from build123d import *

# Parameters (mm, degrees)
BOSS_EXTRUDE2_DEPTH = 1.6
CUT_EXTRUDE3_START  = 1.6
SKETCH1_R           = 0.5
CUT_EXTRUDE3_DEPTH  = 47.684310176
CUT_EXTRUDE4_START  = 1.6
SKETCH3_R           = 1
CUT_EXTRUDE4_DEPTH  = 1.6
FILLET1_R           = 1


with BuildPart() as part:
    # Sketch2 → Boss-Extrude2 (new body)
    with BuildSketch(Plane.XY):
        with BuildLine():
            Line((-16.263194882, -20.445638098), (-23.811184851, -29.934762))
            ThreePointArc((-23.811184851, -29.934762), (0, -38.25), (23.811184851, -29.934762))
            Line((23.811184851, -29.934762), (16.263194882, -20.445638098))
            ThreePointArc((16.263194882, -20.445638098), (0, -26.125), (-16.263194882, -20.445638098))
        make_face()
    extrude(amount=BOSS_EXTRUDE2_DEPTH)

    # Sketch1 → Cut-Extrude3 (cut, through all)
    with BuildSketch(Plane.XY.offset(CUT_EXTRUDE3_START)):
        with Locations((-15.454132619, -23.797277365)):
            Circle(SKETCH1_R)
        with Locations((-12.88198043, -25.282310124)):
            Circle(SKETCH1_R)
        with Locations((-10.168690568, -26.490344602)):
            Circle(SKETCH1_R)
        with Locations((-7.343990405, -27.408145321)):
            Circle(SKETCH1_R)
        with Locations((-4.438827946, -28.025656664)):
            Circle(SKETCH1_R)
        with Locations((-1.485032758, -28.336113049)):
            Circle(SKETCH1_R)
        with Locations((1.485032758, -28.336113049)):
            Circle(SKETCH1_R)
        with Locations((4.438827946, -28.025656664)):
            Circle(SKETCH1_R)
        with Locations((7.343990405, -27.408145321)):
            Circle(SKETCH1_R)
        with Locations((10.168690568, -26.490344602)):
            Circle(SKETCH1_R)
        with Locations((12.88198043, -25.282310124)):
            Circle(SKETCH1_R)
        with Locations((15.454132619, -23.797277365)):
            Circle(SKETCH1_R)
    extrude(amount=-CUT_EXTRUDE3_DEPTH, mode=Mode.SUBTRACT)

    # Sketch3 → Cut-Extrude4 (cut)
    with BuildSketch(Plane.XY.offset(CUT_EXTRUDE4_START)):
        with Locations((-17.6875, -30.635648659)):
            Circle(SKETCH3_R)
        with Locations((17.6875, -30.635648659)):
            Circle(SKETCH3_R)
    extrude(amount=-CUT_EXTRUDE4_DEPTH, mode=Mode.SUBTRACT)

    # Fillet1
    fillet1_edges = [part.edges().sort_by_distance(p)[0] for p in [
        (16.263194882, -20.445638098, 0.8),
        (23.811184851, -29.934762, 0.8),
        (-23.811184851, -29.934762, 0.8),
        (-16.263194882, -20.445638098, 0.8),
    ]]
    fillet(fillet1_edges, radius=FILLET1_R)


solid = part.part
The listing builds one solid part. Answer for the finished solid, in the listing's coordinates (mm). Round coordinates to 2 decimals unless told otherwise and drop trailing zeros. Loops run counter-clockwise (first coordinate to the right, second up) from the corner with the lowest first, then second, coordinate; pieces in that order, holes last. Notation, with made-up numbers: M 62.25,49.5 L 73.25,49.5 A22 cw 73.25,67.5 Z; hole C 83.25,9 d8. An arc over 180 degrees is marked long. Return JSON: item names as keys, results as strings.
Q1. The mould has two halves that part along Y. Classify faces 1 (the face through (-0.35, -38.25, 0.79)), 2 (the face through (-12.99, -25.77, 0.81)), 3 (the face through (16.212, -20.844, 0.811)): released by +Y, released by -Y, zero draft, split by the parting line, or undercut.
Results list:
{"face 1": "released by -Y", "face 2": "undercut", "face 3": "released by +Y"}
Q2. This flat-tipped pin is pushed along its axis until it touches: pin 1 Ø1.8 at (x, y) = (17.69, -30.64) entering from -Z. Where does it stop, or does it pass through?
Results list:
{"pin 1": "passes through"}
Q3. Find section A-A, the plane x = 17.5. Determine the outline of the cut face in (y, z), plus the area to 3 significant figures.
Results list:
{"outline": "M -34.01,0 L -31.62,0 L -31.62,1.6 L -34.01,1.6 Z; M -29.65,0 L -22,0 L -22,1.6 L -29.65,1.6 Z", "area": "16.1 mm2"}
Q4. Find section D-D, the plane x = -3. Determine the outline of the cut face in (y, z), plus the area to 3 significant figures.
Results list:
{"outline": "M -38.13,0 L -25.95,0 L -25.95,1.6 L -38.13,1.6 Z", "area": "19.5 mm2"}
Q5. Find section C-C, the plane y = -35. Determine the outline of the cut face in (x, z), plus the area to 3 significant figures.
Results list:
{"outline": "M -15.43,0 L 15.43,0 L 15.43,1.6 L -15.43,1.6 Z", "area": "49.4 mm2"}
Q6. Find the intervals of material crossed by line 1 along X through (y, z) = (-30, 0.9); line 2 along X through (y, z) = (-27.75, 0.1); line 3 along X through (y, z) = (-30.5, 0.35), in increasing order. Write a range as from..to.
Results list:
{"line 1": "x = -23.37..-18.46, -16.92..16.92, 18.46..23.37", "line 2": "x = -22.07..-7.71, -6.98..-4.86, -4.02..4.02, 4.86..6.98, 7.71..22.07", "line 3": "x = -23.07..-18.68, -16.7..16.7, 18.68..23.07"}
Q7. Find section B-B, the plane z = 0.3. State how many separate pieces and enclosed holes the cut face has, plus the area to 3 significant figures.
Results list:
{"separate pieces": "1", "enclosed holes": "14", "area": "508 mm2"}
